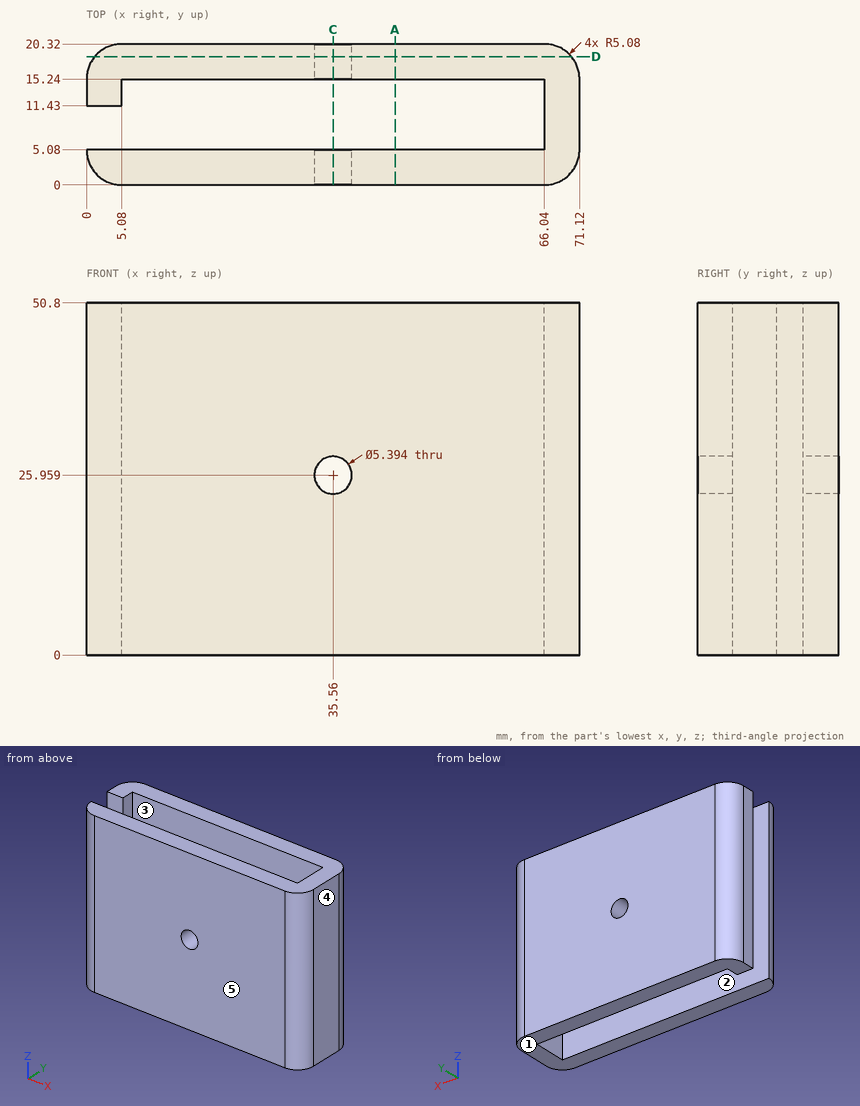
Part print with two shaded views. Sizes in mm from the minimum x, y, z corner. A direction names the side the tool comes from. Round coordinates to 2 decimals unless told otherwise and drop trailing zeros. Loops run counter-clockwise (first coordinate to the right, second up) from the corner with the lowest first, then second, coordinate; pieces in that order, holes last. Notation, with made-up numbers: (11.25, -39.5) - (66.25, -39.5) arc R12 cw to (66.25, -29.5) - close; hole circle Ø5 at (78, 68.5). An arc over 180 degrees is marked (long way). Put each result on its own line as item: value.
1. Two-plate mould, pull along X, no slides. Class the marked faces 3, 4 and 5: released by +X, released by -X, zero draft, split by the parting line, or undercut.
Geometry check:
face 3: undercut
face 4: released by +X
face 5: zero draft
2. Slice it at A-A on x = 44.5. List the corners of the cut face in (y, z), and give its area (3 significant figures).
Geometry check:
outline: (0, 0) - (5.08, 0) - (5.08, 50.8) - (0, 50.8) - close; (15.24, 0) - (20.32, 0) - (20.32, 50.8) - (15.24, 50.8) - close
area: 516 mm²
3. 3-axis set-ups, long thin cutter, end or side, ignore diameter. For the marked faces 1 and 2: which of +Z, -Z, +X, -X, +Y, -Y reach the whole face in a straight line?
Geometry check:
face 1: -Z, +X, -X, +Y, -Y
face 2: +Z, -Z, -X
4. Wall check: line 1 (Y direction, x = 31.5, z = 38); line 2 (Z direction, x = 35.56, y = 3.45); line 3 (X direction, y = 11.75, z = 44.5). Give the ranges that are in metal, low to high.
Geometry check:
line 1: 0 to 5.08, 15.24 to 20.32
line 2: 0 to 23.26, 28.66 to 50.8
line 3: 0 to 5.08, 66.04 to 71.12
5. Pin check, flat tip, straight feed: P1, Ø4.5, axis at x = 35.56, z = 25.96, coming from the -Y side. Stop position of the tip, or through.
Geometry check:
P1: through
6. Slice it at C-C on x = 35.56. List the corners of the cut face in (y, z).
Geometry check:
outline: (0, 0) - (5.08, 0) - (5.08, 23.26) - (0, 23.26) - close; (0, 28.66) - (5.08, 28.66) - (5.08, 50.8) - (0, 50.8) - close; (15.24, 0) - (20.32, 0) - (20.32, 23.26) - (15.24, 23.26) - close; (15.24, 28.66) - (20.32, 28.66) - (20.32, 50.8) - (15.24, 50.8) - close
7. Slice it at D-D on y = 18.5. List the corners of the cut face in (x, z).
Geometry check:
outline: (1.18, 0) - (69.94, 0) - (69.94, 50.8) - (1.18, 50.8) - close; hole circle Ø5.39 at (35.56, 25.96)
